The listing builds one solid part. Answer for the finished solid, in the listing's coordinates (mm). Give positions to 0.01 mm unless a question says otherwise; leave off trailing zeros. Answer as a JSON object with one key per item and string values.
```python
from build123d import *

# Parameters (mm, degrees)
F5_T     = 1
F7_ANGLE = 61.6159971065


# Not quite as in the source:
# - a fillet or chamfer that OpenCascade refuses, or shapes differently, is made with other operations: its cross-section is extruded or revolved along the edge and cut away or added
# - a feature of the source that left no trace in its solid (it failed there, or was rolled back) is left out
# - a shell that OpenCascade refuses in one call is made with other operations: the cavity is built on its own and cut out


with BuildPart() as f1:
    # F0 (on Front) → F1 (revolve)
    with BuildSketch(Plane.XZ):
        Polygon((-42, 4.4344547205), (-42, 0), (0, 0), (0, 3.3141644672), (-0.939540565, 3.3141644672), (-0.939540565, 2.5), (-12.3243089765, 2.5), (-12.3243089765, 3.1194374897), (-13.1681719795, 3.1194374897), (-13.1681719795, 2.5), (-25.396803394, 2.5), (-25.396803394, 3.3141644672), (-28.4831486642, 3.3141644672), (-28.4831486642, 2.5), (-36.2527966499, 2.5), (-39.1136556864, 4.4344547205), align=None)
    revolve(axis=Axis((-21, 0, 0), (1, 0, 0)))

    # F4: fillet of radius 5 on 1 edges, made by hand

    # F4_s1 → F4_t2 (revolve)
    with BuildSketch(Plane.XZ):
        with BuildLine():
            ThreePointArc((-0.939540565, 3.3141644672), (-2.2475981784, 2.7078617683), (-3.6742765472, 2.5))
            Line((-3.6742765472, 2.5), (-0.939540565, 2.5))
            Line((-0.939540565, 2.5), (-0.939540565, 3.3141644672))
        make_face()
    revolve(axis=Axis((-0.939540565, 0, 0), (1, 0, 0)))

    # F5: shell of thickness 1, made by hand


with BuildPart() as f5_core1:
    # F5_t2: copy of F1
    add(f1.part)

    # the walls: a layer under each face that stays
    f5_faces = [f5_core1.faces().sort_by_distance(p)[0] for p in [
        (-40.5568278432, 0, -4.4344547205),
        (-37.6832261682, 0, -3.4672273602),
        (-32.3679726571, 0, -2.5),
        (-28.4831486642, 2.2094429781, -2.2094429781),
        (-26.9399760291, 0, -3.3141644672),
        (-25.396803394, 2.2094429781, 2.2094429781),
        (-19.2824876867, 0, -2.5),
        (-13.1681719795, 2.0796249931, -2.0796249931),
        (-12.746240478, 0, -3.1194374897),
        (-12.3243089765, 2.0796249931, 2.0796249931),
        (-7.9992927619, 0, -2.5),
        (-2.2475981784, 0, -2.7078617683),
        (-0.4697702825, 0, -3.3141644672),
    ]]
    thicken(f5_faces, amount=-F5_T, mode=Mode.SUBTRACT)

    # F5_s3 → F5_t4 (revolve, cut)
    with BuildSketch(Plane.XZ):
        Polygon((-36.2471952097, 2.5182839524), (-36.8129406711, 1.6716047589), (-36.5591549299, 1.5), (-36.2527966499, 1.5), align=None)
    revolve(axis=Axis((-36.2527966499, 0, 0), (1, 0, 0)), mode=Mode.SUBTRACT)

    # F5_s5 → F5_t6 (revolve, cut)
    with BuildSketch(Plane.XZ):
        Polygon((-28.4931486642, 2.51), (-28.4831486642, 1.5), (-27.4831486642, 1.5), (-27.4831486642, 2.5), align=None)
    revolve(axis=Axis((-28.4831486642, 0, 0), (1, 0, 0)), mode=Mode.SUBTRACT)

    # F5_s7 → F5_t8 (revolve, cut)
    with BuildSketch(Plane.XZ):
        Polygon((-25.386803394, 2.51), (-26.396803394, 2.5), (-26.396803394, 1.5), (-25.396803394, 1.5), align=None)
    revolve(axis=Axis((-25.396803394, 0, 0), (1, 0, 0)), mode=Mode.SUBTRACT)

    # F5_s9 → F5_t10 (revolve, cut)
    with BuildSketch(Plane.XZ):
        Polygon((-13.1781719795, 2.51), (-13.1681719795, 1.5), (-12.1681719795, 1.5), (-12.1681719795, 2.5), align=None)
    revolve(axis=Axis((-13.1681719795, 0, 0), (1, 0, 0)), mode=Mode.SUBTRACT)

    # F5_s11 → F5_t12 (revolve, cut)
    with BuildSketch(Plane.XZ):
        Polygon((-12.3143089765, 2.51), (-13.3243089765, 2.5), (-13.3243089765, 1.5), (-12.3243089765, 1.5), align=None)
    revolve(axis=Axis((-12.3243089765, 0, 0), (1, 0, 0)), mode=Mode.SUBTRACT)


with BuildPart() as f1_1:
    add(f1.part)

    # what is left inside the walls is the cavity
    f5_cavity = [f5_core1.part.solids().sort_by_distance(p)[0] for p in [
        (-18.822628, 0, -1.49),
    ]]
    add(f5_cavity, mode=Mode.SUBTRACT)

    # F6 (on Top) → F7 (revolve)
    with BuildSketch(Plane.XY):
        Polygon((-0.2392299093, -68.1274962625), (118.1739337362, 136.1414027413), (-117.9347038269, 136.5557610989), align=None)
    revolve(axis=Axis((0.1196149546, 136.3485819201, 0), (0.9999984601, -0.0017549452, 0)), revolution_arc=F7_ANGLE)


solid = f1_1.part
```
1. Consider line 1 along Z through (x, y) = (-40.85, 0); line 2 along Y through (x, z) = (11, -78); line 3 along Y through (x, z) = (40.5, -19). Determine where each line is inside the solid, lowest interval first.
Verdict:
{"line 1": "z = -4.43 to -3.43, 3.43 to 4.43", "line 2": "y = -31.56 to 94.18", "line 3": "y = 3.5 to 126.01"}
2. The mould has two halves that part along X. Classify faces 1 (the flat face through (-42, 3, 2)), 2 (the conical face through (59.82, 49.28, -50.98)), 3 (the conical face through (-37.068, -0.576, 2.996)): released by +X, released by -X, zero draft, split by the parting line, or undercut.
Verdict:
{"face 1": "released by -X", "face 2": "released by +X", "face 3": "undercut"}
3. Flat-ended cylindrical pins translate along their axes: pin 1 (12 mm diameter, centred on y = 80, z = -47, fed in from -X); pin 2 (5.5 mm diameter, centred on y = 0, z = 0, fed in from -X); pin 3 (8 mm diameter, centred on x = -47.5, z = -41, fed in from +Y). Find the tip coordinate at first contact, or state that the pin passes through.
Verdict:
{"pin 1": "stops at x = -79.06", "pin 2": "stops at x = -40.99", "pin 3": "stops at y = 116.44"}
